Input: dimensioned drawing with shaded views. Units: mm. Origin: part minimum x, y, z. A direction names the side the tool comes from. Round coordinates to 2 decimals unless told otherwise and drop trailing zeros. Loops run counter-clockwise (first coordinate to the right, second up) from the corner with the lowest first, then second, coordinate; pieces in that order, holes last. Notation, with made-up numbers: (-39.5, 10.5) - (-16.5, 10.5) arc R21 cw to (-16.5, 43.5) - close; hole circle Ø11 at (72, -27.75). An arc over 180 degrees is marked (long way). One line per question, with ' | ' between items. Start each with the question number.
1. Cut plane D-D (z = 52.5). Return loops of the section in (x, y), then the cut area to 3 significant figures.
2. Access query for the marked faces 3 and 4. Directions: +Z, -Z, +X, -X, +Y, -Y. A direction counts if a zero-diameter tool reaches every point of the face in a straight line with its end or side. Return the directions, or none.
3. Cut plane B-B (x = 25). Return loops of the section in (y, z).
4. Ray query, line 1 (Y direction, x = 25, z = 5.75); line 2 (Y direction, x = 25.5, z = 27) (3 decimals); line 3 (Y direction, x = 45.5, z = 27.5). Return the intervals inside material, ascending.
5. Pin query (flat end, axial travel): pin 1 (4.5 mm diameter, centred on x = 25, y = 175, fed in from +Z); pin 2 (1 mm diameter, centred on y = 155, z = 28, fed in from -X); pin 3 (10 mm diameter, centred on x = 37, y = 124, fed in from +Z) (3 decimals); pin 4 (1.5 mm diameter, centred on y = 87, z = 31, fed in from -X). Return the tip coordinate at first contact, or that it passes through.
6. Cut plane C-C (y = 47.5). Return loops of the section in (x, z), then the cut area to 3 significant figures.
7. Mould query, pull axis Y, two halves, no side actions, for the marked faces 1 and 2. Classes: pulls with the +Y half, pulls with the -Y half, needs draft (parallel to the pull), parting line crosses it, or undercut.
8. Cut plane A-A (z = 85). Return loops of the section in (x, y).
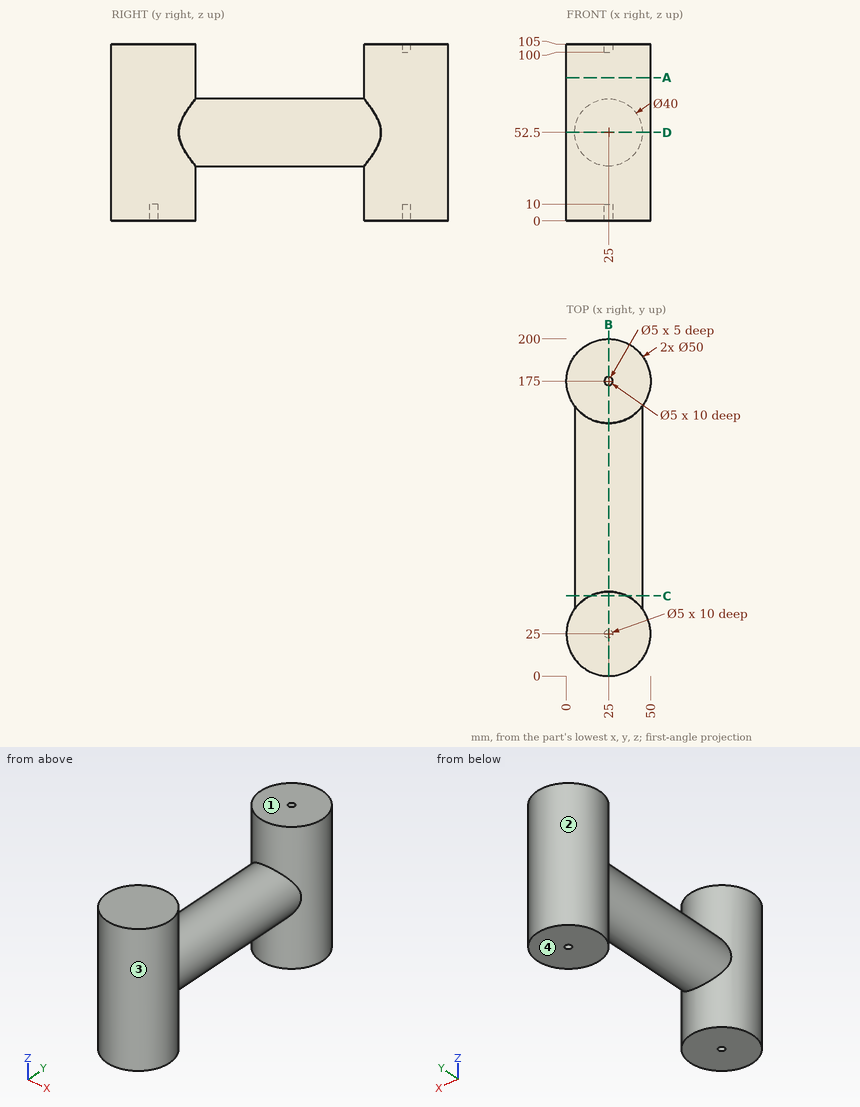
Answers follow:
1) outline: (5, 40) arc R25 ccw (long way) to (45, 40) - (45, 160) arc R25 ccw (long way) to (5, 160) - close | area: 8,170 mm2
2) face 3: none | face 4: -Z, +X, -X, +Y, -Y
3) outline: (0, 0) - (22.5, 0) - (22.5, 10) - (27.5, 10) - (27.5, 0) - (50, 0) - (50, 32.5) - (150, 32.5) - (150, 0) - (172.5, 0) - (172.5, 10) - (177.5, 10) - (177.5, 0) - (200, 0) - (200, 105) - (177.5, 105) - (177.5, 100) - (172.5, 100) - (172.5, 105) - (150, 105) - (150, 72.5) - (50, 72.5) - (50, 105) - (0, 105) - close
4) line 1: y = 0 to 22.5, 27.5 to 50, 150 to 172.5, 177.5 to 200 | line 2: y = 0.005 to 49.995, 150.005 to 199.995 | line 3: y = 10.69 to 39.31, 160.69 to 189.31
5) pin 1: stops at z = 100 | pin 2: stops at x = 9.36 | pin 3: stops at z = 71.235 | pin 4: passes through
6) outline: (14.1, 0) - (35.9, 0) - (35.9, 35.73) arc R20 ccw to (35.9, 69.27) - (35.9, 105) - (14.1, 105) - (14.1, 69.27) arc R20 ccw to (14.1, 35.73) - close | area: 2,720 mm2
7) face 1: needs draft | face 2: undercut
8) outline: circle Ø50 at (25, 25); circle Ø50 at (25, 175)
